The figure shows three views and two pictorial views of one solid part (mm, origin at its lowest corner). Answer the questions. A direction names the side the tool comes from. Give positions to 0.01 mm unless a question says otherwise; leave off trailing zeros. Write each loop counter-clockwise with the first axis right and the second up, starting at its lowest first coordinate (ties: lowest second). Pieces come first, ordered by that corner, then holes. Notation, with made-up numbers: (81, 84.25) -> (99, 84.25) arc R17 cw to (99, 112.25) -> close; hole circle Ø2 at (-20, 85). An arc over 180 degrees is marked (long way). Use a Markdown table: item, result.
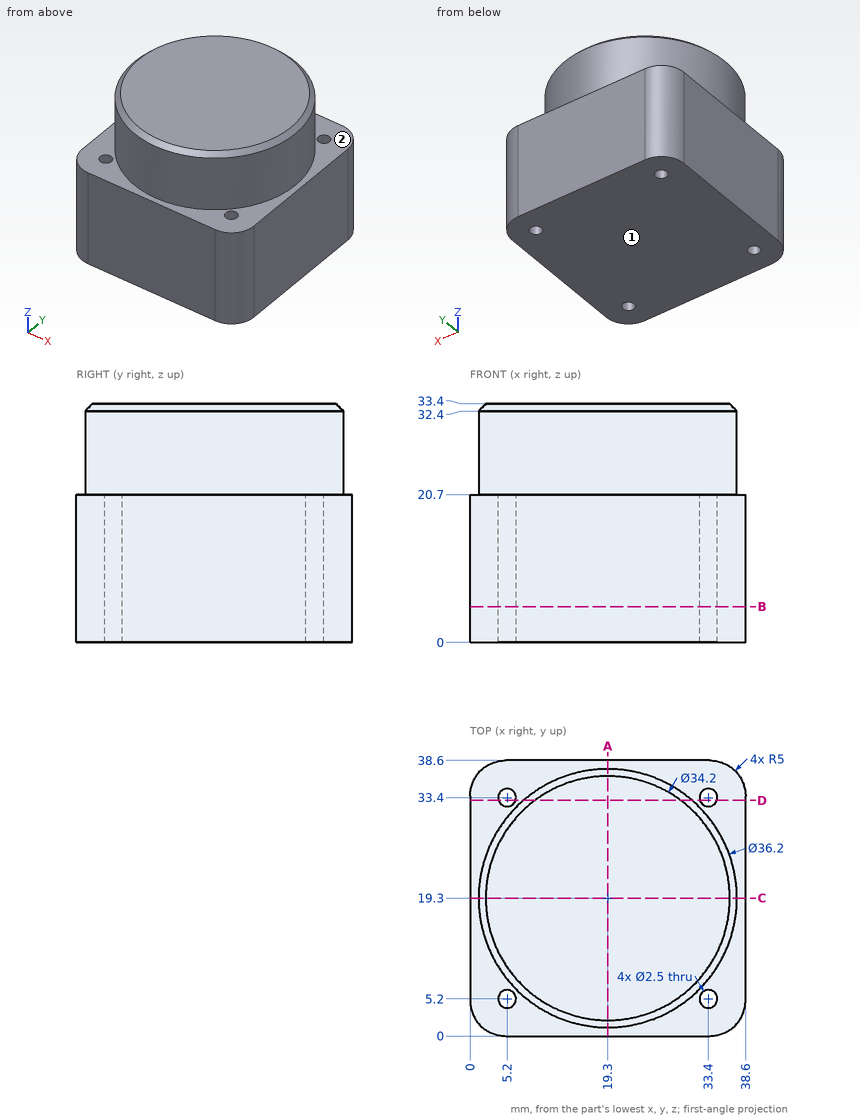
Item 1: A cutting plane is placed at D-D (y = 33). Count the separate pieces of the cut face and the enclosed holes in it, then the cut area to 4 significant figures.
Return value:
| item | result |
|---|---|
| separate pieces | 3 |
| enclosed holes | 0 |
| area | 1,000 mm^2 |
Item 2: A tool of negligible diameter and unlimited length cuts with its end or side. For the marked faces 1 and 2, from which of +Z, -Z, +X, -X, +Y, -Y can it reach the whole face along a straight path? Write none if from no direction.
Return value:
| item | result |
|---|---|
| face 1 | -Z, +X, -X, +Y, -Y |
| face 2 | +Z |
Item 3: A cutting plane is placed at B-B (z = 5). Give the vertices of the cut face in (x, y), then the cut area to 3 significant figures.
Return value:
| item | result |
|---|---|
| outline | (0, 5) arc R5 ccw to (5, 0) -> (33.6, 0) arc R5 ccw to (38.6, 5) -> (38.6, 33.6) arc R5 ccw to (33.6, 38.6) -> (5, 38.6) arc R5 ccw to (0, 33.6) -> close; hole circle Ø2.5 at (5.2, 5.2); hole circle Ø2.5 at (5.2, 33.4); hole circle Ø2.5 at (33.4, 5.2); hole circle Ø2.5 at (33.4, 33.4) |
| area | 1,450 mm^2 |
Item 4: Each of these flat-tipped pins is pushed along its axis until it touches: P1, Ø3, axis at x = 33.4, y = 33.4, coming from the +Z side; P2, Ø1, axis at y = 22.5, z = 22.5, coming from the -X side; P3, Ø12, axis at x = 23, z = 28.5, coming from the +Y side; P4, Ø2, axis at x = 5.2, y = 33.4, coming from the +Z side. Where does it stop, or does it pass through?
Return value:
| item | result |
|---|---|
| P1 | z = 20.7 |
| P2 | x = 1.4 |
| P3 | y = 37.4 |
| P4 | through |
Item 5: Straight lines are drawn through the part: line 1 along X through (y, z) = (33.4, 7.5); line 2 along Y through (x, z) = (34, 2). For each, find the intervals that lie inside material, in ascending order. Write a range as [from, to].
Return value:
| item | result |
|---|---|
| line 1 | [0, 3.95], [6.45, 32.15], [34.65, 38.6] |
| line 2 | [0.02, 4.1], [6.3, 32.3], [34.5, 38.58] |
Item 6: A cutting plane is placed at A-A (x = 19.3). Give the vertices of the cut face in (y, z), then the cut area to 3 significant figures.
Return value:
| item | result |
|---|---|
| outline | (0, 0) -> (38.6, 0) -> (38.6, 20.7) -> (37.4, 20.7) -> (37.4, 32.4) -> (36.4, 33.4) -> (2.2, 33.4) -> (1.2, 32.4) -> (1.2, 20.7) -> (0, 20.7) -> close |
| area | 1,260 mm^2 |
